Can you work these out from the model? Positions are in its coordinate system, mm. Face numbers are marked on the shaded views. A direction names the side the tool comes from. Give positions to 0.01 mm unless a question says otherwise; leave off trailing zeros. Loops run counter-clockwise (first coordinate to the right, second up) from the corner with the lowest first, then second, coordinate; pieces in that order, holes last. Notation, with made-up numbers: (9.25, 89.5) - (47.25, 89.5) arc R20 ccw to (47.25, 106.5) - close; hole circle Ø1 at (-21.5, -7.75). An arc over 180 degrees is marked (long way). Write item = value, one per line.
from build123d import *

# Parameters (mm, degrees)
EXTRUDE_1_DEPTH = 10
EXTRUDE_2_DEPTH = 5
SKETCH_4_W      = 5
SKETCH_4_H      = 8
EXTRUDE_3_DEPTH = 3
CHAMFER_1_SIZE  = 3


# Read off the part's stored shape, not the designer's step: 高级异型孔3, 高级异型孔4
with BuildPart() as part:
    # 草图1 → 凸台-拉伸1 (new body)
    with BuildSketch(Plane(origin=(0, 0, 0), x_dir=(1, 0, 0), z_dir=(0, 1, 0))):
        Polygon((0, 0), (5, -8), (5, 0), (15, 0), (15, -8), (20, 0), (20, 30), (0, 30), align=None)
    extrude(amount=-EXTRUDE_1_DEPTH)

    # 草图2 → 凸台-拉伸2 (add, symmetric)
    with BuildSketch(Plane(origin=(10, 0, 0), x_dir=(0, 0, -1), z_dir=(1, 0, 0))):
        with BuildLine():
            Line((0, 30), (-3, 33))
            Line((-3, 33), (-3, 90))
            Line((-3, 90), (-18, 90))
            Line((-18, 90), (-18, 80))
            ThreePointArc((-18, 80), (-10, 72), (-18, 64))
            Line((-18, 64), (-18, 54))
            Line((-18, 54), (-20, 0))
            Line((-20, 0), (-20, -10))
            Line((-20, -10), (-10, -20))
            Line((-10, -20), (0, -20))
            Line((0, -20), (10, -10))
            Line((10, -10), (0, -10))
            Line((0, -10), (0, 30))
        make_face()
    extrude(amount=EXTRUDE_2_DEPTH, both=True)

    # 草图4 → 凸台-拉伸3 (add)
    with BuildSketch(Plane(origin=(0, 0, 0), x_dir=(1, 0, 0), z_dir=(0, 1, 0))):
        with Locations((2.5, 15)):
            Rectangle(SKETCH_4_W, SKETCH_4_H)
        with Locations((17.5, 15)):
            Rectangle(SKETCH_4_W, SKETCH_4_H)
    extrude(amount=EXTRUDE_3_DEPTH)

    # 高级异型孔3 outline → 高级异型孔3 (revolve, cut)
    with BuildSketch(Plane(origin=(10, 0, -15), x_dir=(1, 0, 0), z_dir=(0, 0, 1))):
        Polygon((0, -10), (3.15, -10), (1.7, -8.55), (1.7, 0), (0, 0), align=None)
    revolve(axis=Axis((10, 0, -15), (0, 1, 0)), mode=Mode.SUBTRACT)

    # 高级异型孔4 outline → 高级异型孔4 (revolve, cut)
    with BuildSketch(Plane(origin=(10, 59, 0), x_dir=(1, 0, 0), z_dir=(0, -1, 0))):
        Polygon((0, 7.008579979), (1.65, 8), (1.65, 18), (0, 18), align=None)
    revolve(axis=Axis((10, 59, 0), (0, 0, 1)), mode=Mode.SUBTRACT)

    # Other 4 2 outline → Other 4 2 (revolve, cut)
    with BuildSketch(Plane(origin=(10, 85, 0), x_dir=(1, 0, 0), z_dir=(0, -1, 0))):
        Polygon((0, 7.008579979), (1.65, 8), (1.65, 18), (0, 18), align=None)
    revolve(axis=Axis((10, 85, 0), (0, 0, 1)), mode=Mode.SUBTRACT)

    # 倒角1
    chamfer_1_edges = [part.edges().sort_by_distance(p)[0] for p in [
        (10, 90, 3),
    ]]
    chamfer(chamfer_1_edges, length=CHAMFER_1_SIZE)


solid = part.part
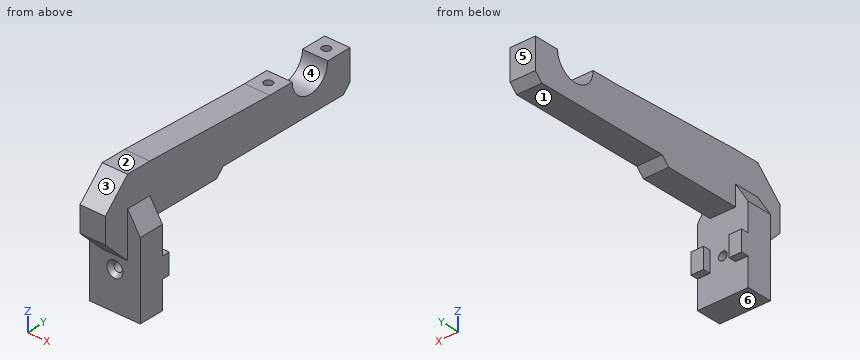
Q1. Imagine slicing it at C-C, the plane z = -23. Write out the boundary of the cut face in (x, y), then the cut area to 3 significant figures.
Output:
outline = (0, -10) - (20, -10) - (20, 0) - (0, 0) - close
area = 200 mm2
Q2. For pin 1 (2.5 mm diameter, centred on x = 10, z = -15, fed in from -Y); pin 2 (11 mm diameter, centred on x = 8, y = 57.5, fed in from +Z); pin 3 (8 mm diameter, centred on x = 9.5, y = 22.5, fed in from -Z); pin 4 (0.9 mm diameter, centred on x = 2, y = 2, fed in from -Z), each with a flat end and sliding along its axis, tell me the tip position at first contact or that it passes through.
Output:
pin_1 = through
pin_2 = 18.07
pin_3 = 0
pin_4 = -19
Q3. Imagine slicing it at B-B, the plane x = 4. Write out the boundary of the cut face in (y, z).
Output:
outline = (-10, -30) - (0, -30) - (0, -19) - (3, -19) - (3, -11) - (0, -11) - (0, 6.4) - (-10, 6.4) - close
Q4. Which directions (+Z, -Z, +X, -X, +Y, -Y) give clear straight access to the entire face, cutting with the end or side of a thin tool? Please do the marked faces 1 and 2.
Output:
face_1 = -Z, +X, -X, +Y
face_2 = +Z, +X, -X, +Y, -Y
Q5. I need wall thicknesses on L1, parallel to Z at x = 10, y = -3.75; L2, parallel to Y at x = 10, z = 13.5; L3, parallel to X at y = 85, z = 10. Which ranges of each line are inside material? Lowest first, please.
Output:
L1 = -30 to -16.7, -13.3 to 20
L2 = -16.5 to 57.35, 60.65 to 65.39, 78.61 to 83.35, 86.65 to 90
L3 = 5 to 8.35, 11.65 to 15
Q6. We'd pull the mould along Y, two halves only. Please class the marked faces 3, 4, 5 and 6: released by +Y, released by -Y, zero draft, split by the parting line, or undercut.
Output:
face_3 = released by -Y
face_4 = undercut
face_5 = released by +Y
face_6 = zero draft
Q7. Imagine slicing it at D-D, the plane y = 72. Write out the boundary of the cut face in (x, z).
Output:
outline = (5, 3) - (15, 3) - (15, 10) - (5, 10) - close
Q8. Imagine slicing it at A-A, the plane y = -4. Write out the boundary of the cut face in (x, z), then the cut area to 3 significant figures.
Output:
outline = (0, -30) - (20, -30) - (20, 0) - (15, 8) - (15, 20) - (5, 20) - (5, 8) - (0, 0) - close; hole circle Ø3.4 at (10, -15)
area = 831 mm2
